```python
from build123d import *

# Parameters (mm, degrees)
F0_W        = 116.1797607577
F0_H        = 190.5
F1_DEPTH    = 304.8
F3_DEPTH    = 401.32
F4_DEPTH    = 942.34
F5_T1_DEPTH = 331.0069513468
F5_T3_DEPTH = 352.1111565483
F5_T5_DEPTH = 464.9612906349
F5_T7_DEPTH = 766.5905156751
F5_T9_DEPTH = 766.5905156751


# Not quite as in the source:
# - a fillet or chamfer that OpenCascade refuses, or shapes differently, is made with other operations: its cross-section is extruded or revolved along the edge and cut away or added


with BuildPart() as f1:
    # F0 (on Top) → F1 (new body)
    with BuildSketch(Plane.XY):
        Polygon((50.8, 190.5), (50.8, 279.4), (-88.9, 279.4), (-88.9, 190.5), (-88.9, 0), (0, 0), (50.8, 0), align=None)
        Polygon((188.6202392423, 231.1629162652), (50.8, 279.4), (50.8, 190.5), (188.6202392423, 190.5), align=None)
        Polygon((-88.9, 190.5), (-88.9, 279.4), (-304.8, 190.5), (-304.8, 0), (-188.6202392423, 0), (-88.9, 0), align=None)
        Polygon((304.8, 190.5), (188.6202392423, 231.1629162652), (188.6202392423, 190.5), align=None)
        with Locations((246.7101196212, 95.25)):
            Rectangle(F0_W, F0_H)
        Polygon((50.8, -190.5), (50.8, 0), (0, 0), (-88.9, 0), (-88.9, -190.5), (-88.9, -279.4), (50.8, -279.4), align=None)
        Polygon((-88.9, -190.5), (-88.9, 0), (-188.6202392423, 0), (-304.8, 0), (-304.8, -190.5), (-88.9, -279.4), align=None)
        with Locations((246.7101196212, -95.25)):
            Rectangle(F0_W, F0_H)
        Polygon((188.6202392423, -190.5), (50.8, -190.5), (50.8, -279.4), (188.6202392423, -231.1629162652), align=None)
        Polygon((304.8, -190.5), (188.6202392423, -190.5), (188.6202392423, -231.1629162652), align=None)
    extrude(amount=F1_DEPTH)

    # F2 (on Front) → F3 (cut)
    with BuildSketch(Plane.XZ):
        Polygon((306.468307972, 307.1446120739), (38.1901785731, 0), (-147.3951488733, -79.8071026802), (42.6088683307, 0), (5.996810738, -19.8390558362), (306.468307972, -19.8390558362), align=None)
    extrude(amount=-F3_DEPTH, mode=Mode.SUBTRACT)

    # F2 (on Front) → F4 (cut)
    with BuildSketch(Plane.XZ):
        Polygon((306.468307972, 307.1446120739), (38.1901785731, 0), (-147.3951488733, -79.8071026802), (42.6088683307, 0), (5.996810738, -19.8390558362), (306.468307972, -19.8390558362), align=None)
    extrude(amount=F4_DEPTH, mode=Mode.SUBTRACT)

    # F5: fillet of radius 47.8312768991 on 8 edges, made by hand

    # F5_s2 → F5_t1 (cut)
    with BuildSketch(Plane.XY.offset(-5.8851483368)):
        with BuildLine():
            ThreePointArc((42.671278796, 279.4), (50.6850979696, 278.7238898597), (58.4723614349, 276.7146734978))
            Line((58.4723614349, 276.7146734978), (50.8, 279.4))
            Line((50.8, 279.4), (42.671278796, 279.4))
        make_face()
        with BuildLine():
            ThreePointArc((58.4723614349, -276.7146734978), (50.6850979696, -278.7238898597), (42.671278796, -279.4))
            Line((42.671278796, -279.4), (50.8, -279.4))
            Line((50.8, -279.4), (58.4723614349, -276.7146734978))
        make_face()
    extrude(amount=F5_T1_DEPTH, mode=Mode.SUBTRACT)

    # F5_s4 → F5_t3 (cut)
    with BuildSketch(Plane.XY.offset(-23.6555782741)):
        with BuildLine():
            ThreePointArc((-97.6495180547, 275.7972572716), (-88.7201117415, 278.4906706018), (-79.4377686903, 279.4))
            Line((-79.4377686903, 279.4), (-88.9, 279.4))
            Line((-88.9, 279.4), (-97.6495180547, 275.7972572716))
        make_face()
        with BuildLine():
            ThreePointArc((-79.4377686903, -279.4), (-88.7201117415, -278.4906706018), (-97.6495180547, -275.7972572716))
            Line((-97.6495180547, -275.7972572716), (-88.9, -279.4))
            Line((-88.9, -279.4), (-79.4377686903, -279.4))
        make_face()
    extrude(amount=F5_T3_DEPTH, mode=Mode.SUBTRACT)

    # F5_s6 → F5_t5 (cut)
    with BuildSketch(Plane.XY.offset(-80.0806453175)):
        with BuildLine():
            ThreePointArc((-304.8, 158.467741873), (-296.7111580821, 185.0829614206), (-275.1804724653, 202.6962760437))
            Line((-275.1804724653, 202.6962760437), (-304.8, 190.5))
            Line((-304.8, 190.5), (-304.8, 158.467741873))
        make_face()
        with BuildLine():
            ThreePointArc((-275.1804724653, -202.6962760437), (-296.7111580821, -185.0829614206), (-304.8, -158.467741873))
            Line((-304.8, -158.467741873), (-304.8, -190.5))
            Line((-304.8, -190.5), (-275.1804724653, -202.6962760437))
        make_face()
    extrude(amount=F5_T5_DEPTH, mode=Mode.SUBTRACT)

    # F5_s8 → F5_t7 (cut)
    with BuildSketch(Plane(origin=(300.5564502803, -105.1947575981, 344.0992172359), x_dir=(-0.3303504247, -0.9438583564, 0), z_dir=(-0.6410735721, 0.2243757502, -0.7339483619))):
        with BuildLine():
            ThreePointArc((-280.4958263449, 79.454688834), (-270.4603992444, 50.1407879029), (-244.5651615788, 33.1275209877))
            Line((-244.5651615788, 33.1275209877), (-280.4958263449, 42.357459379))
            Line((-280.4958263449, 42.357459379), (-280.4958263449, 79.454688834))
        make_face()
    extrude(amount=F5_T7_DEPTH, mode=Mode.SUBTRACT)

    # F5_s10 → F5_t9 (cut)
    with BuildSketch(Plane(origin=(300.5564502803, 105.1947575981, 344.0992172359), x_dir=(0.3303504247, -0.9438583564, 0), z_dir=(-0.6410735721, -0.2243757502, -0.7339483619))):
        with BuildLine():
            ThreePointArc((280.4958263449, 79.454688834), (270.4603992444, 50.1407879029), (244.5651615788, 33.1275209877))
            Line((244.5651615788, 33.1275209877), (280.4958263449, 42.357459379))
            Line((280.4958263449, 42.357459379), (280.4958263449, 79.454688834))
        make_face()
    extrude(amount=F5_T9_DEPTH, mode=Mode.SUBTRACT)


solid = f1.part
```
Geometry: final body of the model. Coordinates: model frame, mm. A direction names the side the tool comes from. Give positions to 0.01 mm unless a question says otherwise; leave off trailing zeros. Loops run counter-clockwise (first coordinate to the right, second up) from the corner with the lowest first, then second, coordinate; pieces in that order, holes last. Notation, with made-up numbers: (-27, -4) -> (6, -4) arc R16 ccw to (6, 22) -> close; hole circle Ø5 at (65.5, 46). An arc over 180 degrees is marked (long way). Return JSON: item names as keys, results as strings.
Item 1: Access query for faces 4 (the flat face through (50.8, -3, 158)), 5 (the cylindrical face through (164.41, -229.29, 160.18)). Directions: +Z, -Z, +X, -X, +Y, -Y. A direction counts if a zero-diameter tool reaches every point of the face in a straight line with its end or side. Return the directions, or none.
Filled in:
{"face 4": "+Z, -Z", "face 5": "-Z, +X, -Y"}
Item 2: Mould query, pull axis X, two halves, no side actions, for faces 1 (the flat face through (112.152, -257.927, 240.167)), 2 (the flat face through (-18, 279.4, 150)), 3 (the flat face through (103, 190.5, 190)). Classes: released by +X, released by -X, zero draft, split by the parting line, or undercut.
Filled in:
{"face 1": "released by +X", "face 2": "zero draft", "face 3": "undercut"}
Item 3: Pin query (flat end, axial travel): P1, Ø1, axis at y = 167.5, z = 97.5, coming from the -X side; P2, Ø2, axis at y = -12, z = 77, coming from the +X side; P3, Ø8, axis at x = -228, z = 165, coming from the -Y side. Return the tip coordinate at first contact, or that it passes through.
Filled in:
{"P1": "x = -304.03", "P2": "x = 50.8", "P3": "y = -223.77"}
Item 4: Section A-A, the plane y = 4.5. Output: boundary loops of the cut face in (x, z).
Filled in:
{"outline": "(-304.8, 0) -> (38.19, 0) -> (50.8, 14.44) -> (50.8, 304.8) -> (-304.8, 304.8) -> close; (188.62, 172.22) -> (304.42, 304.8) -> (188.62, 304.8) -> close"}
Item 5: Line query: line 1 (Y direction, x = 133, z = 257.5); line 2 (Y direction, x = 98.5, z = 136.5) (3 decimals); line 3 (X direction, y = 20, z = 230.5). Output: solid intervals per line, ascending.
Filled in:
{"line 1": "-250.63 to -190.5, 190.5 to 250.63", "line 2": "-262.705 to -190.5, 190.5 to 262.705", "line 3": "-304.8 to 50.8, 188.62 to 239.52"}
Item 6: Section B-B, the plane x = -230. Output: boundary loops of the cut face in (y, z).
Filled in:
{"outline": "(-221.3, 0) -> (221.3, 0) -> (221.3, 304.8) -> (-221.3, 304.8) -> close"}
